from build123d import *

# Parameters (mm, degrees)
F1_DEPTH       = 50
F3_D           = 3.4
F3_DEPTH       = 3
F3_CBORE_D     = 6.5
F3_CBORE_DEPTH = 2
F3_TIP         = 1.0214630523
F2_W           = 6
F2_H           = 1
F4_DEPTH       = 0.7
F5_T4_DEPTH    = 55.1433659759
F5_T9_DEPTH    = 55.1433659759
F5_T14_DEPTH   = 6.1433659759
F5_T19_DEPTH   = 6.1433659759
F5_T24_DEPTH   = 6.1433659759
F5_T29_DEPTH   = 6.1433659759
F6_T1_DEPTH    = 15


# Not quite as in the source:
# - a fillet or chamfer that OpenCascade refuses, or shapes differently, is made with other operations: its cross-section is extruded or revolved along the edge and cut away or added


with BuildPart() as f1:
    # F0 (on Top) → F1 (new body)
    with BuildSketch(Plane.XY):
        Polygon((-5.8, -2.5), (5.8, -2.5), (5.8, 2.5), (3.4, 2.5), (3.4, 1.5), (4.4, 1.5), (4.4, 0.6), (-4.4, 0.6), (-4.4, 1.5), (-3.4, 1.5), (-3.4, 2.5), (-5.8, 2.5), align=None)
    extrude(amount=F1_DEPTH)

    # F3
    with Locations(Plane(origin=(0, 0.6, 0), x_dir=(-1, 0, 0), z_dir=(0, 1, 0))):
        with Locations((0, 30), (0, 20)):
            CounterBoreHole(F3_D / 2, F3_CBORE_D / 2, F3_CBORE_DEPTH, depth=F3_DEPTH)
            with Locations((0, 0, -(F3_DEPTH + F3_TIP / 2))):  # 118° drill point
                Cone(0, F3_D / 2, F3_TIP, mode=Mode.SUBTRACT)

    # F2 (on face) → F4 (join)
    with BuildSketch(Plane(origin=(0, 0.6, 0), x_dir=(-1, 0, 0), z_dir=(0, 1, 0))):
        with Locations((0, 49.5)):
            Rectangle(F2_W, F2_H)
        with Locations((0, 0.5)):
            Rectangle(F2_W, F2_H)
    extrude(amount=F4_DEPTH)

    # F5: chamfer of 1 on 6 edges, made by hand


with BuildPart() as f5_tool2:
    # F5_s3 → F5_t4 (new body)
    with BuildSketch(Plane.XY.offset(-2.571682988)):
        Polygon((3.4, 2.5), (4.4, 1.5), (3.4, 1.5), align=None)
    extrude(amount=F5_T4_DEPTH)

    split(bisect_by=Plane.YZ.offset(4.4), keep=Keep.BOTTOM)


with BuildPart() as f1_1:
    add(f1.part)

    # F5_t1: cut F5_tool2
    add(f5_tool2.part, mode=Mode.SUBTRACT)


with BuildPart() as f5_tool7:
    # F5_s8 → F5_t9 (new body)
    with BuildSketch(Plane.XY.offset(-2.571682988)):
        Polygon((-4.4, 1.5), (-3.4, 2.5), (-3.4, 1.5), align=None)
    extrude(amount=F5_T9_DEPTH)

    split(bisect_by=Plane.YZ.offset(-4.4), keep=Keep.TOP)


with BuildPart() as f1_2:
    add(f1_1.part)

    # F5_t6: cut F5_tool7
    add(f5_tool7.part, mode=Mode.SUBTRACT)


with BuildPart() as f5_tool12:
    # F5_s13 → F5_t14 (new body)
    with BuildSketch(Plane.XY.offset(-2.571682988)):
        Polygon((-3, 0.3), (-2, 1.3), (-3, 1.3), align=None)
    extrude(amount=F5_T14_DEPTH)

    split(bisect_by=Plane.XZ.offset(-0.6), keep=Keep.BOTTOM)


with BuildPart() as f1_3:
    add(f1_2.part)

    # F5_t11: cut F5_tool12
    add(f5_tool12.part, mode=Mode.SUBTRACT)


with BuildPart() as f5_tool17:
    # F5_s18 → F5_t19 (new body)
    with BuildSketch(Plane.XY.offset(3.571682988)):
        Polygon((3, 0.3), (2, 1.3), (3, 1.3), align=None)
    extrude(amount=-F5_T19_DEPTH)

    split(bisect_by=Plane.XZ.offset(-0.6), keep=Keep.BOTTOM)


with BuildPart() as f1_4:
    add(f1_3.part)

    # F5_t16: cut F5_tool17
    add(f5_tool17.part, mode=Mode.SUBTRACT)


with BuildPart() as f5_tool22:
    # F5_s23 → F5_t24 (new body)
    with BuildSketch(Plane.XY.offset(52.571682988)):
        Polygon((3, 0.3), (2, 1.3), (3, 1.3), align=None)
    extrude(amount=-F5_T24_DEPTH)

    split(bisect_by=Plane.XZ.offset(-0.6), keep=Keep.BOTTOM)


with BuildPart() as f1_5:
    add(f1_4.part)

    # F5_t21: cut F5_tool22
    add(f5_tool22.part, mode=Mode.SUBTRACT)


with BuildPart() as f5_tool27:
    # F5_s28 → F5_t29 (new body)
    with BuildSketch(Plane.XY.offset(46.428317012)):
        Polygon((-3, 0.3), (-2, 1.3), (-3, 1.3), align=None)
    extrude(amount=F5_T29_DEPTH)

    split(bisect_by=Plane.XZ.offset(-0.6), keep=Keep.BOTTOM)


with BuildPart() as f1_6:
    add(f1_5.part)

    # F5_t26: cut F5_tool27
    add(f5_tool27.part, mode=Mode.SUBTRACT)

    # F6: fillet of radius 2 on 4 edges, made by hand

    # F6_s2 → F6_t1 (cut)
    with BuildSketch(Plane.XZ.offset(-7.5)):
        with BuildLine():
            ThreePointArc((5.8, 48), (5.2142135624, 49.4142135624), (3.8, 50))
            Line((3.8, 50), (5.8, 50))
            Line((5.8, 50), (5.8, 48))
        make_face()
        with BuildLine():
            ThreePointArc((-3.8, 50), (-5.2142135624, 49.4142135624), (-5.8, 48))
            Line((-5.8, 48), (-5.8, 50))
            Line((-5.8, 50), (-3.8, 50))
        make_face()
        with BuildLine():
            ThreePointArc((-3.8, 0), (-5.2142135624, 0.5857864376), (-5.8, 2))
            Line((-5.8, 2), (-5.8, 0))
            Line((-5.8, 0), (-3.8, 0))
        make_face()
        with BuildLine():
            ThreePointArc((5.8, 2), (5.2142135624, 0.5857864376), (3.8, 0))
            Line((3.8, 0), (5.8, 0))
            Line((5.8, 0), (5.8, 2))
        make_face()
    extrude(amount=F6_T1_DEPTH, mode=Mode.SUBTRACT)


solid = f1_6.part
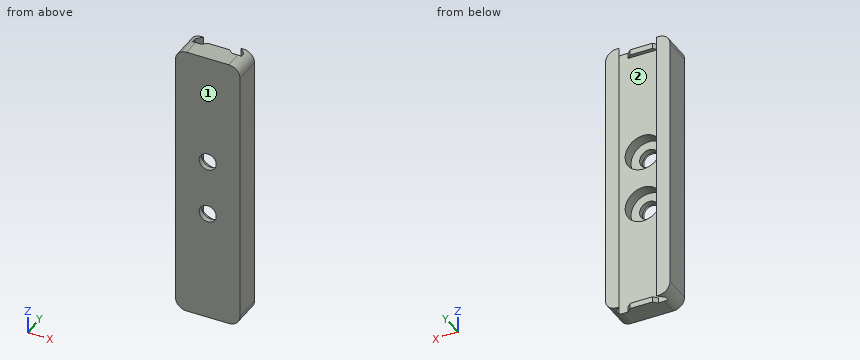
Verification items for the finished model (mm, model axes). Face numbers are marked on the shaded views. Round coordinates to 2 decimals unless told otherwise and drop trailing zeros. Write each loop counter-clockwise with the first axis right and the second up, starting at its lowest first coordinate (ties: lowest second). Pieces come first, ordered by that corner, then holes.
(1) Depth check by flat-ended pin: pin 1 Ø2.5 at (x, z) = (0, 20) entering from -Y. Enter the tip coordinate at first touch or a pass-through.
Returned:
pin 1: passes through
(2) Material ranges on line 1 (Z direction, x = -0.25, y = 0.15); line 2 (Y direction, x = -3, z = 6); line 3 (X direction, y = -1.85, z = 20), recorded low to high.
Returned:
line 1: z = 0 to 16.76, 23.24 to 26.76, 33.24 to 50
line 2: y = -2.5 to 0.6
line 3: x = -5.8 to -1.7, 1.7 to 5.8
(3) Section check C-C (x = 0). Enter the section's corners in (y, z).
Returned:
outline: (-2.5, 0) - (1.3, 0) - (1.3, 1) - (0.6, 1) - (0.6, 16.75) - (-1.4, 16.75) - (-1.4, 18.3) - (-2.4, 18.3) - (-2.5, 18.47) - close; (-2.5, 21.53) - (-2.4, 21.7) - (-1.4, 21.7) - (-1.4, 23.25) - (0.6, 23.25) - (0.6, 26.75) - (-1.4, 26.75) - (-1.4, 28.3) - (-2.4, 28.3) - (-2.5, 28.47) - close; (-2.5, 31.53) - (-2.4, 31.7) - (-1.4, 31.7) - (-1.4, 33.25) - (0.6, 33.25) - (0.6, 49) - (1.3, 49) - (1.3, 50) - (-2.5, 50) - close
(4) Section check B-B (y = -0.5). Enter the section's corners in (x, z), plus the area to 3 significant figures.
Returned:
outline: (-5.8, 2) arc R2 ccw to (-3.8, 0) - (3.8, 0) arc R2 ccw to (5.8, 2) - (5.8, 48) arc R2 ccw to (3.8, 50) - (-3.8, 50) arc R2 ccw to (-5.8, 48) - close; hole circle Ø6.5 at (0, 20); hole circle Ø6.5 at (0, 30)
area: 510 mm2
(5) Mould release check, pull along Y, two halves, no side actions. Record for the marked faces 1 and 2: pulls with the +Y half, pulls with the -Y half, needs draft (parallel to the pull), parting line crosses it, or undercut.
Returned:
face 1: pulls with the -Y half
face 2: undercut
(6) Section check D-D (z = 42.5). Enter the section's corners in (x, y).
Returned:
outline: (-5.8, -2.5) - (5.8, -2.5) - (5.8, 2.5) - (3.4, 2.5) - (4.4, 1.5) - (4.4, 0.6) - (-4.4, 0.6) - (-4.4, 1.5) - (-3.4, 2.5) - (-5.8, 2.5) - close
(7) Section check A-A (z = 30). Enter the section's corners in (x, y).
Returned:
outline: (-5.8, -2.5) - (-1.53, -2.5) - (-1.7, -2.4) - (-1.7, -1.4) - (-3.25, -1.4) - (-3.25, 0.6) - (-4.4, 0.6) - (-4.4, 1.5) - (-3.4, 2.5) - (-5.8, 2.5) - close; (1.53, -2.5) - (5.8, -2.5) - (5.8, 2.5) - (3.4, 2.5) - (4.4, 1.5) - (4.4, 0.6) - (3.25, 0.6) - (3.25, -1.4) - (1.7, -1.4) - (1.7, -2.4) - close
